For this review, take the finished solid that the model builds, in its own axes (mm). A direction names the side the tool comes from. Coordinates: 2 decimals unless noted, no trailing zeros. Write each loop counter-clockwise with the first axis right and the second up, starting at its lowest first coordinate (ties: lowest second). Pieces come first, ordered by that corner, then holes. Notation, with made-up numbers: M -36.75,75 L 9.25,75 A27 ccw 9.25,107 Z; hole C 6,-29 d9. An arc over 180 degrees is marked long. One line per question, with ' | ' between items.
Autodesk Inventor part; units mm, degrees
ref_plane "YZ Plane" through (0, 0, 0) normal (1, 0, 0) x (0, 1, 0)
ref_plane "XZ Plane" through (0, 0, 0) normal (0, 1, 0) x (-1, 0, 0)
ref_plane "XY Plane" through (0, 0, 0) normal (0, 0, 1) x (1, 0, 0)
sketch "Эскиз1" plane through (0, 0, 0) normal (0, 0, 1) x (1, 0, 0)
  line L0 (-173.0013, 292.0364) -> (-157.0013, 292.0364)
  line L1 (-157.0013, 292.0364) -> (-157.0013, 246.0364)
  line L2 (-157.0013, 246.0364) -> (-173.0013, 246.0364)
  line L3 (-173.0013, 246.0364) -> (-173.0013, 292.0364)
  circle A0 centre (-165.0013, 284.0364) radius 1.5
  circle A1 centre (-165.0013, 254.0364) radius 1.5
  line L4 (-165.0013, 284.0364) -> (-165.0013, 254.0364) construction
  line L5 (-157.0013, 292.0364) -> (-145.0013, 292.0364)
  line L6 (-145.0013, 292.0364) -> (-145.0013, 280.5364)
  line L7 (-145.0013, 280.5364) -> (-157.0013, 280.5364) construction
  line L8 (-157.0013, 280.5364) -> (-157.0013, 292.0364)
  line L9 (-157.0013, 269.0364) -> (-145.0013, 269.0364) construction
  line L10 (-145.0013, 269.0364) -> (-145.0013, 257.5364)
  line L11 (-145.0013, 257.5364) -> (-157.0013, 257.5364) construction
  line L12 (-157.0013, 257.5364) -> (-157.0013, 269.0364)
  line L13 (-145.0013, 292.0364) -> (-129.0013, 292.0364)
  line L14 (-129.0013, 292.0364) -> (-129.0013, 246.0364)
  line L15 (-129.0013, 246.0364) -> (-145.0013, 246.0364)
  line L16 (-145.0013, 246.0364) -> (-145.0013, 292.0364)
  line L17 (-145.0013, 254.7807) -> (-145.0013, 246.0364)
  line L18 (-145.0013, 246.0364) -> (-157.0013, 246.0364)
  line L19 (-157.0013, 246.0364) -> (-157.0013, 254.7807)
  line L20 (-157.0013, 280.3864) -> (-145.0013, 280.3864)
  line L21 (-157.0013, 269.1864) -> (-145.0013, 269.1864)
  line L22 (-157.0013, 257.3864) -> (-145.0013, 257.3864)
  point P0 (0, 0)
  dimension "d0" = 3
  dimension "d1" = 3
  dimension "d2" = 8
  dimension "d3" = 8
  dimension "d4" = 30
  dimension "d5" = 46
  dimension "d6" = 8
  dimension "d7" = 8
  dimension "d8" = 46
  dimension "d9" = 16
  dimension "d10" = 44
  dimension "d11" = 12
  dimension "d12" = 16
  dimension "d13" = 11.5
  dimension "d14" = 11.5
  dimension "d15" = 11.5
  dimension "d16" = 11.5
  dimension "d17" = 0.15
  dimension "d18" = 0.15
  dimension "d19" = 0.15
extrude "Выдавливание1" add sketch "Эскиз1" along normal blind 4 contours L0 L1 L2 L3
extrude "Выдавливание2" add sketch "Эскиз1" along normal blind 10 contours L1 L22 L16 L18 | L20 L16 L21 L1
sketch "Эскиз2" plane through (-173.0013, 246.0364, 0) normal (0, -1, 0) x (1, 0, 0)
  line L0 (28, 0) -> (16, 0)
  line L1 (22, 0) -> (22, 10) construction
  circle A0 centre (22, 5) radius 1.5
  line L2 (16, 10) -> (28, 10)
  circle A1 centre (22, 5) radius 5
  line L3 (28, 10) -> (16, 10)
  line L4 (22, 10) -> (28, 10)
  line L5 (28, 0) -> (28, 10)
  line L6 (28, 10) -> (28, 0)
  line L7 (28, 0) -> (22, 0)
  line L8 (16, 0) -> (28, 0)
  arc A2 (22, 0) -> (22, 10) centre (22, 5) ccw
  line L9 (0, 4) -> (16, 4)
  line L10 (16, 4) -> (17, 4)
  line L11 (17, 4) -> (17, 5)
  line L12 (16, 4) -> (16, 10)
  line L13 (16, 4) -> (16, 10)
  arc A3 (22, 10) -> (17, 5) centre (22, 5) ccw
  line L14 (16, 10) -> (22, 10)
  line L15 (16, 10) -> (28, 10)
  point P0 (173.0013, 0)
  dimension "d24" = 3
extrude "Выдавливание3" cut sketch "Эскиз2" against normal blind 50 contours L0 A1 L2 L5 | L11 L10 L12 L2 A1
extrude "Выдавливание4" cut sketch "Эскиз2" against normal blind 50 contours A0
fillet "Сопряжение1" radius 10 2 edges at (-173.0013, 292.0364, 2) (-173.0013, 246.0364, 2)
fillet "Сопряжение2" radius 1 5 edges at (-160.0013, 292.0364, 4) (-173.0013, 269.0364, 4) (-170.0724, 248.9654, 4) (-159.5013, 246.0364, 4) (-170.0724, 289.1075, 4)
fillet "Сопряжение3" radius 0.5 24 edges at (-157.0013, 291.7435, 3.7071) (-157.0013, 292.0364, 1.5) (-157.0013, 285.7114, 4) (-154.0013, 280.3864, 0) (-156.0013, 280.3864, 4.5) (-147.4658, 280.3864, 8.5355) (-156.5013, 269.1864, 4) (-156.0013, 269.1864, 4.5) (-154.0013, 269.1864, 0) (-147.4658, 269.1864, 8.5355) (-157.0013, 263.2864, 4) (-156.5013, 257.3864, 4) (-154.0013, 257.3864, 0) (-156.0013, 257.3864, 4.5) (-147.4658, 257.3864, 8.5355) (-156.0013, 246.0364, 3.5) (-156.0013, 246.0364, 4.5) (-157.0013, 246.0364, 0) (-170.0724, 248.9654, 0) (-173.0013, 269.0364, 0) (-170.0724, 289.1075, 0) (-160.0013, 292.0364, 0) (-147.4658, 246.0364, 8.5355) (-156.5013, 280.3864, 4)
chamfer "Фаска1" distance 1.5 angle 45 2 edges at (-166.5013, 254.0364, 4) (-166.5013, 284.0364, 4)
properties part number "петля"
1) Machinability: for faces 4 (the flat face through (-153, 246.036, 4)), 5 (the flat face through (-153, 280.386, 5)), 6 (the flat face through (-156.001, 274.7, 4.5)), 7 (the conical face through (-167, 284, 3)), 8 (the cylindrical face through (-159.3, 246.32, 3.7)), which of the approach directions +Z, -Z, +X, -X, +Y, -Y give a long, thin tool a straight path to every point of the face, cutting with its end or side? Answer none if there is none.
Responses:
face 4: +Z, -Z, +X, -X, -Y | face 5: +Z, -Z, +X, +Y | face 6: +Z, -X, +Y, -Y | face 7: +Z | face 8: +Z, -X, -Y
2) We need section A-A on y = 271. State the section outline as (x, z) points, then the cut area to 3 significant figures.
Responses:
outline: M -173,0.5 A0.5 ccw -172.5,0 L -151,0 A5 ccw long -156,5 L -156,4 L -172,4 A1 ccw -173,3 Z; hole C -151,5 d3 | area: 145 mm^2
3) We need section B-B on x = -161.25. State the section outline as (y, z) points, then the cut area to 3 significant figures.
Responses:
outline: M 246.04,0.5 A0.5 ccw 246.54,0 L 291.54,0 A0.5 ccw 292.04,0.5 L 292.04,3 A1 ccw 291.04,4 L 247.04,4 A1 ccw 246.04,3 Z | area: 183 mm^2
4) The part is to be moulded in two halves that separate along Z. For faces 1 (the conical face through (-167, 254, 3)), 2 (the flat face through (-153, 269.186, 5)), 3 (the cylindrical face through (-152.5, 274.71, 5.07)), say which applies: +Z half, -Z half, draft (parallel to the pull), parting line (faces both ways), or undercut.
Responses:
face 1: +Z half | face 2: draft | face 3: undercut
5) We need section D-D on z = 1.5. State how many separate pieces and enclosed holes the cut face has, then the cut area to 3 significant figures.
Responses:
separate pieces: 1 | enclosed holes: 2 | area: 894 mm^2
6) We need section C-C on y = 264. State the section outline as (x, z) points.
Responses:
outline: M -173,0.5 A0.5 ccw -172.5,0 L -157,0 L -157,3.5 A0.5 ccw -157.5,4 L -172,4 A1 ccw -173,3 Z
7) To check wall thickness, follow line 1 along Y through (x, z) = (-147.5, 4.25); line 2 along Y through (x, z) = (-171.5, 3.5); line 3 along X through (y, z) = (264, 2.75). State the ranges of each line that lie inside material, in increasing order. Write a range as [from, to].
Responses:
line 1: [246.04, 257.39], [269.19, 280.39] | line 2: [251.03, 287.05] | line 3: [-173, -157]
8) Insertion check: pin 1 Ø12 at (x, y) = (-159, 262.5) entering from -Z; pin 2 Ø1 at (y, z) = (284.5, 1.5) entering from +X; pin 3 Ø5 at (x, y) = (-165, 254.04) entering from +Z; pin 4 Ø0.6 at (y, z) = (252, 4.5) entering from -X. Each pin has a flat end and moves straight along its axis. Give the tip position at first contact, or say it passes through.
Responses:
pin 1: z = 0 | pin 2: x = -157 | pin 3: z = 3.5 | pin 4: x = -156
